Check sheet for the modelled part. Datum: model origin and axes. Units: mm. A direction names the side the tool comes from. Give positions to 0.01 mm unless a question says otherwise; leave off trailing zeros. Order: outer loops, then holes, each group sorted by start corner. A loop starts at its lowest first (then second) coordinate and runs counter-clockwise, first axis right, second up.
Item 1: Sectioned sample at D-D on x = -38.5. Record the boundary of the cut face in (y, z).
Item 2: Release check for a two-part mould opening along Z. For faces 1 (the flat face through (-35.022, 97.272, 34.296)), 2 (the flat face through (0.43, 58.31, 46.76)), 3 (the flat face through (-51.5, 121, 25)) record: released by +Z, released by -Z, zero draft, split by the parting line, or undercut.
Item 3: Gauge pin test, flat ends, axial feed: P1, Ø8, axis at y = 27, z = 26, coming from the +X side; P2, Ø8, axis at y = 80.5, z = 46, coming from the -X side; P3, Ø2, axis at y = 125, z = 53.5, coming from the -X side. Record the tip position at first contact, or that the pin passes through.
Item 4: Material ranges on line 1 along Z through (x, y) = (0.5, 143); line 2 along Z through (x, y) = (27, 126.5); line 3 along X through (y, z) = (74.5, 44), recorded low to high.
Item 5: Sectioned sample at A-A on x = 28.5. Record the boundary of the cut face in (y, z), and give its area (3 significant figures).
Item 6: Sectioned sample at B-B on y = 95. Record the boundary of the cut face in (x, z).
Item 7: Sectioned sample at C-C on z = 53.5. Record the boundary of the cut face in (x, y), and give its area (3 significant figures).
Item 8: Access from +Z, -Z, +X, -X, +Y, -Y to the whole of each face (thin tool, end or side, straight path). Record for faces 4 (the flat face through (-31, 68, 42)), 5 (the flat face through (31, 68, 42)), 6 (the flat face through (25.08, 73.13, 40.53)).
from build123d import *

# Parameters (mm, degrees)
F1_DEPTH = 51.5
F2_DEPTH = 19
F3_DEPTH = 31
F5_DEPTH = 200
F7_DEPTH = 200


with BuildPart() as f1:
    # F0 (on Right) → F1 (new body, symmetric)
    with BuildSketch(Plane.YZ):
        Polygon((0, 3), (0, 0), (200, 0), (200, 65), (192.702703, 65), align=None)
    extrude(amount=F1_DEPTH, both=True)

    # F0 (on Right) → F2 (join, symmetric)
    with BuildSketch(Plane.YZ):
        Polygon((0, 17), (0, 3), (192.702703, 65), (149.189189, 65), align=None)
    extrude(amount=F2_DEPTH, both=True)

    # F0 (on Right) → F3 (join, symmetric)
    with BuildSketch(Plane.YZ):
        Polygon((0, 28), (0, 17), (149.189189, 65), (115, 65), align=None)
    extrude(amount=F3_DEPTH, both=True)

    # F4 (on Front) → F5 (cut)
    with BuildSketch(Plane.XZ):
        with BuildLine():
            Line((-51.5, 0), (0, 0))
            Line((0, 0), (0, 2))
            ThreePointArc((0, 2), (-25.76941, 1.499812), (-51.5, 0))
        make_face()
        with BuildLine():
            Line((0, 2), (0, 0))
            Line((0, 0), (51.5, 0))
            ThreePointArc((51.5, 0), (25.76941, 1.499812), (0, 2))
        make_face()
    extrude(amount=-F5_DEPTH, mode=Mode.SUBTRACT)

    # F6 (on Front) → F7 (cut)
    with BuildSketch(Plane.XZ):
        with BuildLine():
            ThreePointArc((0, 65), (25.76941, 64.499812), (51.5, 63))
            Line((51.5, 63), (51.5, 65))
            Line((51.5, 65), (0, 65))
        make_face()
        with BuildLine():
            Line((-51.5, 65), (-51.5, 63))
            ThreePointArc((-51.5, 63), (-25.76941, 64.499812), (0, 65))
            Line((0, 65), (-51.5, 65))
        make_face()
    extrude(amount=-F7_DEPTH, mode=Mode.SUBTRACT)


solid = f1.part
Report:
1. outline: (0, 0.88) - (200, 0.88) - (200, 63.88) - (189.23, 63.88) - (0, 3) - close
2. face 1: undercut
2. face 2: released by +Z
2. face 3: zero draft
3. P1: stops at x = 31
3. P2: stops at x = -31
3. P3: stops at x = -19
4. line 1: z = 2 to 65
4. line 2: z = 1.45 to 43.7, 57.7 to 64.45
4. line 3: x = -31 to 31
5. outline: (0, 1.39) - (200, 1.39) - (200, 64.39) - (190.8, 64.39) - (0, 3) - close; (0, 17) - (147.29, 64.39) - (113.1, 64.39) - (0, 28) - close
5. area: 8,180 mm2
6. outline: (-51.5, 0) arc R664.06 cw to (0, 2) arc R664.06 cw to (51.5, 0) - (51.5, 33.57) - (19, 33.57) - (19, 47.57) - (31, 47.57) - (31, 58.57) - (-31, 58.57) - (-31, 47.57) - (-19, 47.57) - (-19, 33.57) - (-51.5, 33.57) - close
7. outline: (-51.5, 156.96) - (-19, 156.96) - (-19, 113.45) - (-31, 113.45) - (-31, 79.26) - (31, 79.26) - (31, 113.45) - (19, 113.45) - (19, 156.96) - (51.5, 156.96) - (51.5, 200) - (-51.5, 200) - close
7. area: 8,210 mm2
8. face 4: +Z, -X, -Y
8. face 5: +Z, +X, -Y
8. face 6: +X
